Autodesk Inventor part; units mm, degrees
ref_plane "Work Plane7" through (0, 0, 0) normal (0, 0, -1) x (-1, 0, 0)
ref_plane "YZ Plane" through (0, 0, 0) normal (1, 0, 0) x (0, 1, 0)
ref_plane "XZ Plane" through (0, 0, 0) normal (0, 1, 0) x (-1, 0, 0)
sketch "Sketch2" plane through (0, 0, 0) normal (0, 0, 1) x (1, 0, 0)
  circle A0 centre (2.5, 0) radius 1.5
  circle A1 centre (-2.5, 0) radius 1.5
  arc A2 (-1.9231, 1.3846) -> (1.9231, 1.3846) centre (0, 6) ccw
  arc A3 (1.9231, -1.3846) -> (-1.9231, -1.3846) centre (0, -6) ccw
  circle A4 centre (2.5, 0) radius 0.75
  circle A5 centre (-2.5, 0) radius 0.75
  point P0 (0, 0)
  dimension "d0" = 3
  dimension "d1" = 3
  dimension "d2" = 6
  dimension "d3" = 6
  dimension "d4" = 2.5
  dimension "d5" = 2.5
  dimension "d6" = 1.5
  dimension "d7" = 1.5
extrude "Extrusion2" add sketch "Sketch2" along normal blind 0.8
ref_plane "Work Plane7" through (0, 0, 0) normal (0, 0, -1) x (-1, 0, 0)
sketch "Sketch9" plane through (0, 0, 0) normal (0, 0, -1) x (-1, 0, 0)
  arc A0 (1.9231, -1.3846) -> (-1.9231, -1.3846) centre (0, -6) ccw
  arc A1 (1.9231, -1.3846) -> (1.9231, 1.3846) centre (2.5, 0) ccw
  arc A2 (-1.9231, 1.3846) -> (1.9231, 1.3846) centre (0, 6) ccw
  arc A3 (-1.9231, 1.3846) -> (-1.9231, -1.3846) centre (-2.5, 0) ccw
  circle A4 centre (-2.5, 0) radius 0.75
  circle A5 centre (2.5, 0) radius 0.75
  circle A6 centre (-2.5, 0) radius 0.75
  point P0 (0, 0)
extrude "Extrusion8" add sketch "Sketch9" along normal blind 2.5 and the other way blind 1 contours A4
mirror "Mirror7" about plane through (0, 0, 0) normal (1, 0, 0) of "Extrusion8"
mirror "Mirror8" about plane through (-2.5, 0, -2.5) normal (0, 0, -1) of "Extrusion2", "Extrusion8", "Mirror7"
equation "\"d1\" = d0"
equation "\"d7\" = d6"
properties part number "chain ink_outer"
Can you work these out from the model? Positions are in its coordinate system, mm. A direction names the side the tool comes from. Round coordinates to 2 decimals unless told otherwise and drop trailing zeros. Loops run counter-clockwise (first coordinate to the right, second up) from the corner with the lowest first, then second, coordinate; pieces in that order, holes last.
Item 1: If we mould it in two halves opening along Z, with no side actions, what happens to faces 1 (the cylindrical face through (3.095, 0.456, -2.465)), 2 (the flat face through (0, 0, -5)), 3 (the cylindrical face through (-4, 0, -5.4)), 4 (the flat face through (3, 0, 1))? For each: +Z half, -Z half, draft (parallel to the pull), parting line (faces both ways), or undercut.
Item 2: Suppose I cut it at B-B, the plane x = -2.5. Write out the boundary of the cut face in (y, z), then the cut area to 3 significant figures.
Item 3: Please list where these lines run through material, in increasing order: L1, parallel to Z at x = -0.75, y = -0.5; L2, parallel to X at y = 0.05, z = -3.5; L3, parallel to Y at x = -2.25, z = -1.
Item 4: Suppose I cut it at C-C, the plane z = -1. Write out the boundary of the cut face in (x, y).
Item 5: Will these pins go through, and if not, where does the flat tip stop? pin 1 Ø1 at (y, z) = (1, -4) entering from -X; pin 2 Ø1 at (x, z) = (-3, -2) entering from +Y; pin 3 Ø2 at (x, z) = (0, -3.5) entering from +Y.
Item 6: Which directions (+Z, -Z, +X, -X, +Y, -Y) give clear straight access to the entire face, cutting with the end or side of a thin tool? Please do faces 5 (the flat face through (0, 0, 0)), 6 (the cylindrical face through (4, 0, -5.4)), 7 (the flat face through (0, 0, -5.8)), 8 (the flat face through (0, 0, 0.8)), 9 (the flat face through (2, 0, -6)).
Reported:
1. face 1: undercut
1. face 2: undercut
1. face 3: draft
1. face 4: +Z half
2. outline: (-1.5, -5.8) - (-0.75, -5.8) - (-0.75, -6) - (0.75, -6) - (0.75, -5.8) - (1.5, -5.8) - (1.5, -5) - (0.75, -5) - (0.75, 0) - (1.5, 0) - (1.5, 0.8) - (0.75, 0.8) - (0.75, 1) - (-0.75, 1) - (-0.75, 0.8) - (-1.5, 0.8) - (-1.5, 0) - (-0.75, 0) - (-0.75, -5) - (-1.5, -5) - close
2. area: 12.9 mm2
3. L1: z = -5.8 to -5, 0 to 0.8
3. L2: x = -3.25 to -1.75, 1.75 to 3.25
3. L3: y = -0.71 to 0.71
4. outline: circle Ø1.5 at (-2.5, 0); circle Ø1.5 at (2.5, 0)
5. pin 1: stops at x = -3.06
5. pin 2: stops at y = 0.75
5. pin 3: passes through
6. face 5: none
6. face 6: +Z, -Z
6. face 7: -Z
6. face 8: +Z
6. face 9: -Z, +X, -X, +Y, -Y
